```python
from build123d import *

# Parameters (mm, degrees)
SKETCH1_R           = 6
BOSS_EXTRUDE1_DEPTH = 10
SKETCH2_R           = 9.5
BOSS_EXTRUDE2_DEPTH = 1
BOSS_EXTRUDE3_DEPTH = 11
SKETCH4_R           = 9.5
BOSS_EXTRUDE4_DEPTH = 1
SKETCH5_R           = 4
CUT_EXTRUDE1_DEPTH  = 27.636441204
SKETCH6_R           = 2
CUT_EXTRUDE2_DEPTH  = 27.636441204


with BuildPart() as part:
    # Sketch1 → Boss-Extrude1 (new body)
    with BuildSketch(Plane(origin=(0, 0, 0), x_dir=(0, 0, -1), z_dir=(1, 0, 0))):
        Circle(SKETCH1_R)
    extrude(amount=BOSS_EXTRUDE1_DEPTH)

    # Sketch2 → Boss-Extrude2 (add)
    with BuildSketch(Plane(origin=(10, 0, 0), x_dir=(0, 0, -1), z_dir=(1, 0, 0))):
        Circle(SKETCH2_R)
    extrude(amount=BOSS_EXTRUDE2_DEPTH)

    # Sketch3 → Boss-Extrude3 (add)
    with BuildSketch(Plane(origin=(11, 0, 0), x_dir=(0, 0, -1), z_dir=(1, 0, 0))):
        with BuildLine():
            Line((-0.982460567, 7.768118899), (-1.311725835, 6.366268557))
            ThreePointArc((-1.311725835, 6.366268557), (-2.008610463, 6.181867356), (-2.680790278, 5.921432554))
            Line((-2.680790278, 5.921432554), (-3.771158432, 6.862016036))
            ThreePointArc((-3.771158432, 6.862016036), (-4.602358525, 6.334603066), (-5.360813022, 5.707064372))
            Line((-5.360813022, 5.707064372), (-4.803207262, 4.379406352))
            ThreePointArc((-4.803207262, 4.379406352), (-5.258610463, 3.82060414), (-5.64933562, 3.214810577))
            Line((-5.64933562, 3.214810577), (-7.084323087, 3.334856278))
            ThreePointArc((-7.084323087, 3.334856278), (-7.446772523, 2.419603066), (-7.69151711, 1.46610523))
            Line((-7.69151711, 1.46610523), (-6.46002677, 0.719759772))
            ThreePointArc((-6.46002677, 0.719759772), (-6.5, 0), (-6.46002677, -0.719759772))
            Line((-6.46002677, -0.719759772), (-7.69151711, -1.46610523))
            ThreePointArc((-7.69151711, -1.46610523), (-7.446772523, -2.419603066), (-7.084323087, -3.334856278))
            Line((-7.084323087, -3.334856278), (-5.64933562, -3.214810577))
            ThreePointArc((-5.64933562, -3.214810577), (-5.258610463, -3.82060414), (-4.803207262, -4.379406352))
            Line((-4.803207262, -4.379406352), (-5.360813022, -5.707064372))
            ThreePointArc((-5.360813022, -5.707064372), (-4.602358525, -6.334603066), (-3.771158432, -6.862016036))
            Line((-3.771158432, -6.862016036), (-2.680790278, -5.921432554))
            ThreePointArc((-2.680790278, -5.921432554), (-2.008610463, -6.181867356), (-1.311725835, -6.366268557))
            Line((-1.311725835, -6.366268557), (-0.982460567, -7.768118899))
            ThreePointArc((-0.982460567, -7.768118899), (0, -7.83), (0.982460567, -7.768118899))
            Line((0.982460567, -7.768118899), (1.311725835, -6.366268557))
            ThreePointArc((1.311725835, -6.366268557), (2.008610463, -6.181867356), (2.680790278, -5.921432554))
            Line((2.680790278, -5.921432554), (3.771158432, -6.862016036))
            ThreePointArc((3.771158432, -6.862016036), (4.602358525, -6.334603066), (5.360813022, -5.707064372))
            Line((5.360813022, -5.707064372), (4.803207262, -4.379406352))
            ThreePointArc((4.803207262, -4.379406352), (5.258610463, -3.82060414), (5.64933562, -3.214810577))
            Line((5.64933562, -3.214810577), (7.084323087, -3.334856278))
            ThreePointArc((7.084323087, -3.334856278), (7.446772523, -2.419603066), (7.69151711, -1.46610523))
            Line((7.69151711, -1.46610523), (6.46002677, -0.719759772))
            ThreePointArc((6.46002677, -0.719759772), (6.5, 0), (6.46002677, 0.719759772))
            Line((6.46002677, 0.719759772), (7.69151711, 1.46610523))
            ThreePointArc((7.69151711, 1.46610523), (7.446772523, 2.419603066), (7.084323087, 3.334856278))
            Line((7.084323087, 3.334856278), (5.64933562, 3.214810577))
            ThreePointArc((5.64933562, 3.214810577), (5.258610463, 3.82060414), (4.803207262, 4.379406352))
            Line((4.803207262, 4.379406352), (5.360813022, 5.707064372))
            ThreePointArc((5.360813022, 5.707064372), (4.602358525, 6.334603066), (3.771158432, 6.862016036))
            Line((3.771158432, 6.862016036), (2.680790278, 5.921432554))
            ThreePointArc((2.680790278, 5.921432554), (2.008610463, 6.181867356), (1.311725835, 6.366268557))
            Line((1.311725835, 6.366268557), (0.982460567, 7.768118899))
            ThreePointArc((0.982460567, 7.768118899), (0, 7.83), (-0.982460567, 7.768118899))
        make_face()
    extrude(amount=BOSS_EXTRUDE3_DEPTH)

    # Sketch4 → Boss-Extrude4 (add)
    with BuildSketch(Plane(origin=(22, 0, 0), x_dir=(0, 0, -1), z_dir=(1, 0, 0))):
        Circle(SKETCH4_R)
    extrude(amount=BOSS_EXTRUDE4_DEPTH)

    # Sketch5 → Cut-Extrude1 (cut, through all)
    with BuildSketch(Plane.ZY):
        Circle(SKETCH5_R)
    extrude(amount=-CUT_EXTRUDE1_DEPTH, mode=Mode.SUBTRACT)

    # Sketch6 → Cut-Extrude2 (cut, through all)
    with BuildSketch(Plane(origin=(0, 0, 0), x_dir=(1, 0, 0), z_dir=(0, 1, 0))):
        with Locations(Location((5, 0, 0), (0, 0, 270))):
            Circle(SKETCH6_R)
    extrude(amount=-CUT_EXTRUDE2_DEPTH, mode=Mode.SUBTRACT)


solid = part.part
```
Verification items for the finished model (mm, model axes). A direction names the side the tool comes from. Give positions to 0.01 mm unless a question says otherwise; leave off trailing zeros. Order: outer loops, then holes, each group sorted by start corner. A loop starts at its lowest first (then second) coordinate and runs counter-clockwise, first axis right, second up. Notation, with made-up numbers: (34, 1) -> (72, 1) arc R24 ccw to (72, 15) -> close; hole circle Ø3 at (30, 50.5). An arc over 180 degrees is marked (long way). One line per item, written item: value.
(1) Draft check along Y on faces 1 (the face through (16.423, 6.398, -3.234)), 2 (the face through (16.4, 0, -6.5)), 3 (the face through (22.49, -8.43, -4.38)), 4 (the face through (16.42, -3.83, -5.25)). Enter one of: pulls with the +Y half, pulls with the -Y half, needs draft (parallel to the pull), parting line crosses it, or undercut.
Final values:
face 1: pulls with the +Y half
face 2: undercut
face 3: parting line crosses it
face 4: undercut
(2) Sectioned sample at C-C on z = -3.25. Record the cut outline in (x, y), then the cut area to 3 significant figures.
Final values:
outline: (0, -5.04) -> (10, -5.04) -> (10, -8.93) -> (11, -8.93) -> (11, -6.41) -> (22, -6.41) -> (22, -8.93) -> (23, -8.93) -> (23, -2.33) -> (0, -2.33) -> close; (0, 2.33) -> (23, 2.33) -> (23, 8.93) -> (22, 8.93) -> (22, 6.41) -> (11, 6.41) -> (11, 8.93) -> (10, 8.93) -> (10, 5.04) -> (0, 5.04) -> close
area: 170 mm^2
(3) Gauge pin test, flat ends, axial feed: pin 1 (2 mm diameter, centred on x = 11, z = -5, fed in from +Y); pin 2 (5 mm diameter, centred on x = 5, z = 0, fed in from +Y); pin 3 (5 mm diameter, centred on x = 3, y = 5, fed in from -Z). Record the tip position at first contact, or that the pin passes through.
Final values:
pin 1: y = 8.62
pin 2: y = 6
pin 3: z = -5.45
(4) Scan lines: line 1 along X through (y, z) = (-4.95, 0); line 2 along Y through (x, z) = (7.25, 0); line 3 along Y through (x, z) = (17, -5.25). Record each from-to range of solid material in increasing order. Write a range as [from, to].
Final values:
line 1: [0, 3], [7, 23]
line 2: [-6, -4], [4, 6]
line 3: [-5.81, -5.44], [-3.83, 3.83], [5.44, 5.81]
(5) Tool access check on faces 5 (the face through (16.423, -5.053, -5.086)), 6 (the face through (16.423, 7.077, 1.145)), 7 (the face through (16.423, 2.433, 7.442)). Record the directions out of +Z, -Z, +X, -X, +Y, -Y that give a thin tool (end or side, any length) a straight path to the whole face; none if there is none.
Final values:
face 5: -Z
face 6: +Y
face 7: +Z, +Y
(6) Sectioned sample at A-A on y = 0. Record the cut outline in (x, z).
Final values:
outline: (0, -6) -> (10, -6) -> (10, -9.5) -> (11, -9.5) -> (11, -6.5) -> (22, -6.5) -> (22, -9.5) -> (23, -9.5) -> (23, -4) -> (0, -4) -> close; (0, 4) -> (23, 4) -> (23, 9.5) -> (22, 9.5) -> (22, 6.5) -> (11, 6.5) -> (11, 9.5) -> (10, 9.5) -> (10, 6) -> (0, 6) -> close
(7) Sectioned sample at D-D on y = 5. Record the cut outline in (x, z), then the cut area to 3 significant figures.
Final values:
outline: (0, -3.32) -> (10, -3.32) -> (10, -8.08) -> (11, -8.08) -> (11, -5.06) -> (22, -5.06) -> (22, -8.08) -> (23, -8.08) -> (23, 8.08) -> (22, 8.08) -> (22, 5.06) -> (11, 5.06) -> (11, 8.08) -> (10, 8.08) -> (10, 3.32) -> (0, 3.32) -> close
area: 210 mm^2
(8) Sectioned sample at B-B on z = 0. Record the cut outline in (x, y), then the cut area to 3 significant figures.
Final values:
outline: (0, -6) -> (3, -6) -> (3, -4) -> (0, -4) -> close; (0, 4) -> (23, 4) -> (23, 9.5) -> (22, 9.5) -> (22, 7.83) -> (11, 7.83) -> (11, 9.5) -> (10, 9.5) -> (10, 6) -> (0, 6) -> close; (7, -6) -> (10, -6) -> (10, -9.5) -> (11, -9.5) -> (11, -7.83) -> (22, -7.83) -> (22, -9.5) -> (23, -9.5) -> (23, -4) -> (7, -4) -> close
area: 138 mm^2
